```python
from build123d import *

# Parameters (mm, degrees)
SKETCH_1_R      = 1.6
EXTRUDE_1_DEPTH = 2.5
EXTRUDE_START   = 2.5
SKETCH_1_2_R    = 1.6
EXTRUDE_2_DEPTH = 1.5
FILLET_1_R      = 1
FILLET_2_R      = 1
FILLET_3_R      = 0.75


with BuildPart() as part:
    # Эскиз1 → Бобышка-Вытянуть1 (new body)
    with BuildSketch(Plane.XY):
        with BuildLine():
            Line((-26.000019619, -52.3500154), (26.000019619, -52.3500154))
            ThreePointArc((26.000019619, -52.3500154), (28.828446744, -53.521588275), (30.000019619, -56.3500154))
            Line((30.000019619, -56.3500154), (30.000019619, -74.161976935))
            ThreePointArc((30.000019619, -74.161976935), (0, -80), (-30.000019619, -74.161976935))
            Line((-30.000019619, -74.161976935), (-30.000019619, -56.3500154))
            ThreePointArc((-30.000019619, -56.3500154), (-28.828446744, -53.521588275), (-26.000019619, -52.3500154))
        make_face()
        with Locations((-20, -68)):
            Circle(SKETCH_1_R, mode=Mode.SUBTRACT)
        with Locations(Location((20, -68, 0), (0, 0, 180))):
            Circle(SKETCH_1_R, mode=Mode.SUBTRACT)
        with BuildLine():
            Line((-26.000019619, -53.3500154), (2.649996038, -53.3500154))
            ThreePointArc((2.649996038, -53.3500154), (4.771316381, -54.228695057), (5.649996038, -56.3500154))
            Line((5.649996038, -56.3500154), (5.649996038, -63.999979818))
            Line((5.649996038, -63.999979818), (-29.000019619, -63.999979818))
            Line((-29.000019619, -63.999979818), (-29.000019619, -56.3500154))
            ThreePointArc((-29.000019619, -56.3500154), (-28.121339962, -54.228695057), (-26.000019619, -53.3500154))
        make_face(mode=Mode.SUBTRACT)
    extrude(amount=EXTRUDE_1_DEPTH)

    # Эскиз1<2> → Бобышка-Вытянуть2 (add)
    with BuildSketch(Plane.XY.offset(EXTRUDE_START)):
        with BuildLine():
            Line((-26.000019619, -52.3500154), (26.000019619, -52.3500154))
            ThreePointArc((26.000019619, -52.3500154), (28.828446744, -53.521588275), (30.000019619, -56.3500154))
            Line((30.000019619, -56.3500154), (30.000019619, -74.161976935))
            ThreePointArc((30.000019619, -74.161976935), (0, -80), (-30.000019619, -74.161976935))
            Line((-30.000019619, -74.161976935), (-30.000019619, -56.3500154))
            ThreePointArc((-30.000019619, -56.3500154), (-28.828446744, -53.521588275), (-26.000019619, -52.3500154))
        make_face()
        with Locations((-20, -68)):
            Circle(SKETCH_1_2_R, mode=Mode.SUBTRACT)
        with Locations(Location((20, -68, 0), (0, 0, 180))):
            Circle(SKETCH_1_2_R, mode=Mode.SUBTRACT)
    extrude(amount=EXTRUDE_2_DEPTH)

    # Скругление1
    fillet_1_edges = [part.edges().sort_by_distance(p)[0] for p in [
        (5.649996038, -63.999979818, 1.25),
        (-29.000019619, -63.999979818, 1.25),
    ]]
    fillet(fillet_1_edges, radius=FILLET_1_R)

    # Скругление2
    fillet_2_edges = [part.edges().sort_by_distance(p)[0] for p in [
        (30.000019619, -65.255996167, 4),
        (28.828446744, -53.521588275, 4),
        (0, -52.3500154, 4),
        (-28.828446744, -53.521588275, 4),
        (-30.000019619, -65.255996167, 4),
    ]]
    fillet(fillet_2_edges, radius=FILLET_2_R)

    # Скругление3
    # the kernel refuses this fillet: 0.75 mm, written as the material it takes off along each edge
    with BuildSketch(Plane(origin=(-30.000019619, -74.161976935, -1.274451591), x_dir=(0, 1, 0), z_dir=(0, 0, 1))) as fillet_3_piece_1:
        with BuildLine():
            CenterArc((0.507385413, -0.75), FILLET_3_R, 90, 68.34077611)
            ThreePointArc((-0.189661195, -0.473185934), (-0.095207506, -0.236441895), (0, 0))
            Line((0, 0), (0.507385413, 0))
        make_face()
    extrude(amount=5.548903182, mode=Mode.SUBTRACT)
    with BuildSketch(Plane(origin=(30.000019619, -74.161976935, -1.274451591), x_dir=(-0.9282148055127167, -0.3720447215416308, 0), z_dir=(0, 0, 1))) as fillet_3_piece_2:
        with BuildLine():
            CenterArc((0.50739104, -0.749996193), FILLET_3_R, 89.817447948, 68.34077611)
            Line((-0.188770065, -0.470962652), (0, 0))
            ThreePointArc((0, 0), (0.254890318, 0.000406058), (0.509780636, 0))
        make_face()
    extrude(amount=5.548903182, mode=Mode.SUBTRACT)


solid = part.part
```
Work out the finished part from the listing and answer in its coordinate system (mm). A direction names the side the tool comes from. Round coordinates to 2 decimals unless told otherwise and drop trailing zeros. Loops run counter-clockwise (first coordinate to the right, second up) from the corner with the lowest first, then second, coordinate; pieces in that order, holes last. Notation, with made-up numbers: M 52,-19 L 79,-19 A15 ccw 79,1 Z; hole C 48,73 d2. An arc over 180 degrees is marked long. One line per question, with ' | ' between items.
Q1. Consider line 1 along X through (y, z) = (-68, 2.7); line 2 along X through (y, z) = (-58.75, 0.95); line 3 along X through (y, z) = (-67, 2.1). Determine where each line is inside the solid, lowest interval first. Write a range as from..to.
Conclusion:
line 1: x = -30..-21.6, -18.4..18.4, 21.6..30 | line 2: x = -30..-29, 5.65..30 | line 3: x = -30..-21.25, -18.75..18.75, 21.25..30
Q2. Each of these flat-tipped pins is pushed along its axis until it touches: pin 1 Ø1.5 at (x, z) = (14.5, 3.5) entering from -Y; pin 2 Ø1.9 at (x, y) = (20, -68) entering from +Z; pin 3 Ø1 at (x, z) = (6.5, 2.5) entering from -Y; pin 4 Ø11.5 at (x, y) = (-13, -61) entering from -Z. Where does it stop, or does it pass through?
Conclusion:
pin 1: stops at y = -78.81 | pin 2: passes through | pin 3: stops at y = -79.77 | pin 4: stops at z = 0
Q3. Find section D-D, the plane z = 1.1. Give the vertices of the cut face in (x, y).
Conclusion:
outline: M -30,-73.65 A0.75 ccw -29.53,-74.35 A80 ccw 29.53,-74.35 A0.75 ccw 30,-73.65 L 30,-56.35 A4 ccw 26,-52.35 L -26,-52.35 A4 ccw -30,-56.35 Z; hole M -29,-63 A1 ccw -28,-64 L 4.65,-64 A1 ccw 5.65,-63 L 5.65,-56.35 A3 ccw 2.65,-53.35 L -26,-53.35 A3 ccw -29,-56.35 Z; hole C -20,-68 d3.2; hole C 20,-68 d3.2
Q4. Find section A-A, the plane y = -68. Give the vertices of the cut face in (x, z).
Conclusion:
outline: M -30,0 L -21.6,0 L -21.6,4 L -29,4 A1 ccw -30,3 Z; M -18.4,0 L 18.4,0 L 18.4,4 L -18.4,4 Z; M 21.6,0 L 30,0 L 30,3 A1 ccw 29,4 L 21.6,4 Z
Q5. The mould has two halves that part along Y. Classify faces 3 (the cylindrical face through (4.75, -54.21, 1.23)), 4 (the flat face through (0, -52.35, 1)), 5 (the flat face through (-30, -65, 1)): +Y half, -Y half, draft (parallel to the pull), parting line (faces both ways), or undercut.
Conclusion:
face 3: undercut | face 4: +Y half | face 5: draft
Q6. Find section C-C, the plane x = -20. Give the vertices of the cut face in (y, z), then the cut area to 3 significant figures.
Conclusion:
outline: M -77.46,0 L -69.6,0 L -69.6,4 L -77.46,4 Z; M -66.4,0 L -64,0 L -64,2.5 L -53.35,2.5 L -53.35,0 L -52.35,0 L -52.35,3 A1 ccw -53.35,4 L -66.4,4 Z | area: 60.8 mm2
Q7. Find section B-B, the plane y = -59. Give the vertices of the cut face in (x, z), then the cut area to 3 significant figures.
Conclusion:
outline: M -30,0 L -29,0 L -29,2.5 L 5.65,2.5 L 5.65,0 L 30,0 L 30,3 A1 ccw 29,4 L -29,4 A1 ccw -30,3 Z | area: 153 mm2
Q8. A tool of negligible diameter and unlimited length cuts with its end or side. For faces 1 (the cylindrical face through (-28.14, -54.25, 1.23)), 2 (the cylindrical face through (29.715, -65.582, 3.699)), from which of +Z, -Z, +X, -X, +Y, -Y can it reach the whole face along a straight path? Write none if from no direction.
Conclusion:
face 1: -Z | face 2: +Z, +X, +Y, -Y
